Drawing for the job (mm, zero at the part's lowest x, y, z). A direction names the side the tool comes from. Give positions to 0.01 mm unless a question says otherwise; leave off trailing zeros. Loops run counter-clockwise (first coordinate to the right, second up) from the corner with the lowest first, then second, coordinate; pieces in that order, holes last. Notation, with made-up numbers: (65.25, 57) - (105.25, 57) arc R7 ccw to (105.25, 68) - close; hole circle Ø6 at (6, 16.5). An arc over 180 degrees is marked (long way). Return JSON: item names as keys, results as strings. Group by question number.
1) Slice it at D-D (y = 20.75). Count the separate pieces of the cut face and the enclosed holes in it, and give its area (3 significant figures).
2) Slice it at C-C (z = 10.75). List the corners of the cut face in (x, y).
3) Slice it at A-A (x = 23). List the corners of the cut face in (y, z), and give its area (3 significant figures).
4) Drop a flat-ended pin along its axis: pin 1 (1.1 mm diameter, centred on x = 53.5, y = 18.5, fed in from +Z). Give the stop position or say it passes through.
5) Mould opens along Y. For the marked faces 1, 2 and 3 say: released by +Y, released by -Y, zero draft, split by the parting line, or undercut.
6) Drill centre lines: probe 1 along X at (y, z) = (7.25, 6); probe 2 along Y at (x, z) = (29, 6); probe 3 along Y at (x, z) = (16, 9.5). Where is each one in solid material? Low to high. Write a range as from..to.
7) Slice it at B-B (y = 11.5). List the corners of the cut face in (x, z).
8) 3-axis set-ups, long thin cutter, end or side, ignore diameter. For the marked faces 4 and 5: which of +Z, -Z, +X, -X, +Y, -Y reach the whole face in a straight line?
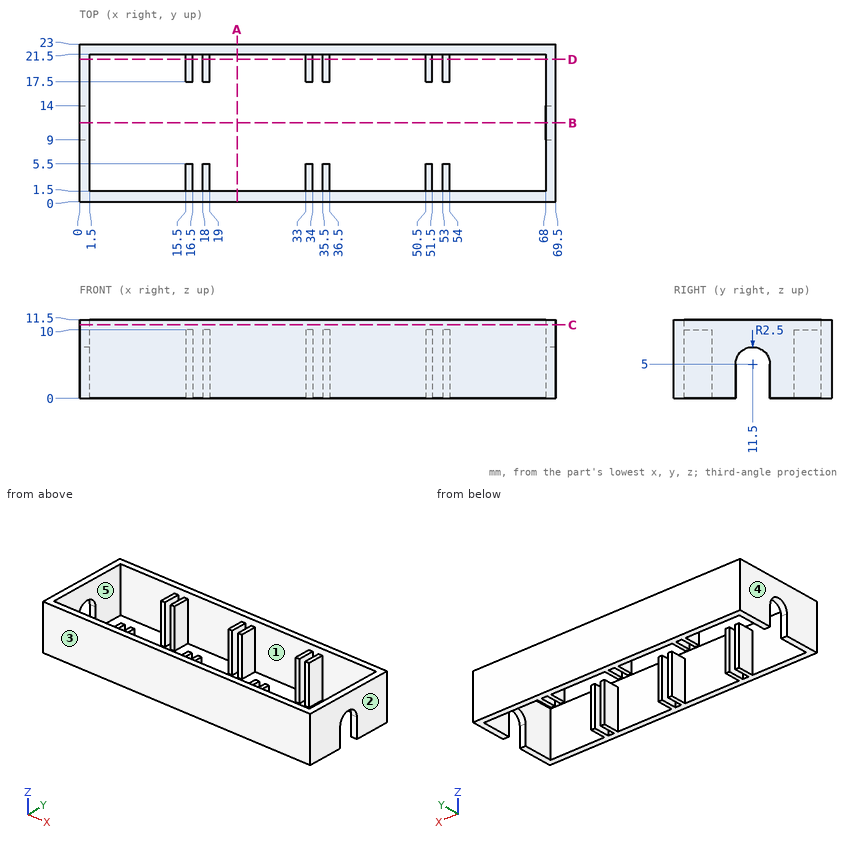
Results:
{
 "1": {"separate pieces": "8", "enclosed holes": "0", "area": "94.5 mm2"},
 "2": {"outline": "(0, 0) - (69.5, 0) - (69.5, 23) - (0, 23) - close; hole (1.5, 1.5) - (68, 1.5) - (68, 21.5) - (1.5, 21.5) - close"},
 "3": {"outline": "(0, 0) - (1.5, 0) - (1.5, 11.5) - (0, 11.5) - close; (21.5, 0) - (23, 0) - (23, 11.5) - (21.5, 11.5) - close", "area": "34.5 mm2"},
 "4": {"pin 1": "z = 10"},
 "5": {"face 1": "undercut", "face 2": "zero draft", "face 3": "released by -Y"},
 "6": {"probe 1": "0..1.5, 68..69.5", "probe 2": "0..1.5, 21.5..23", "probe 3": "0..5.5, 17.5..23"},
 "7": {"outline": "(0, 7.5) - (1.5, 7.5) - (1.5, 11.5) - (0, 11.5) - close; (68, 7.5) - (69.5, 7.5) - (69.5, 11.5) - (68, 11.5) - close"},
 "8": {"face 4": "+Z, -Z, -X, +Y, -Y", "face 5": "+Z, -Z"}
}
